Study the drawing (mm; zero at the part's minimum x, y, z) and answer. Give positions to 0.01 mm unless a question says otherwise; leave off trailing zeros. Write each loop counter-clockwise with the first axis right and the second up, starting at its lowest first coordinate (ties: lowest second). Pieces come first, ordered by that corner, then holes. Notation, with made-up numbers: (12, -6) - (57, -6) arc R17 ccw to (57, 3) - close; hole circle Ø11 at (76.25, 57). An arc over 180 degrees is marked (long way). Answer as CSV lines item,"result".
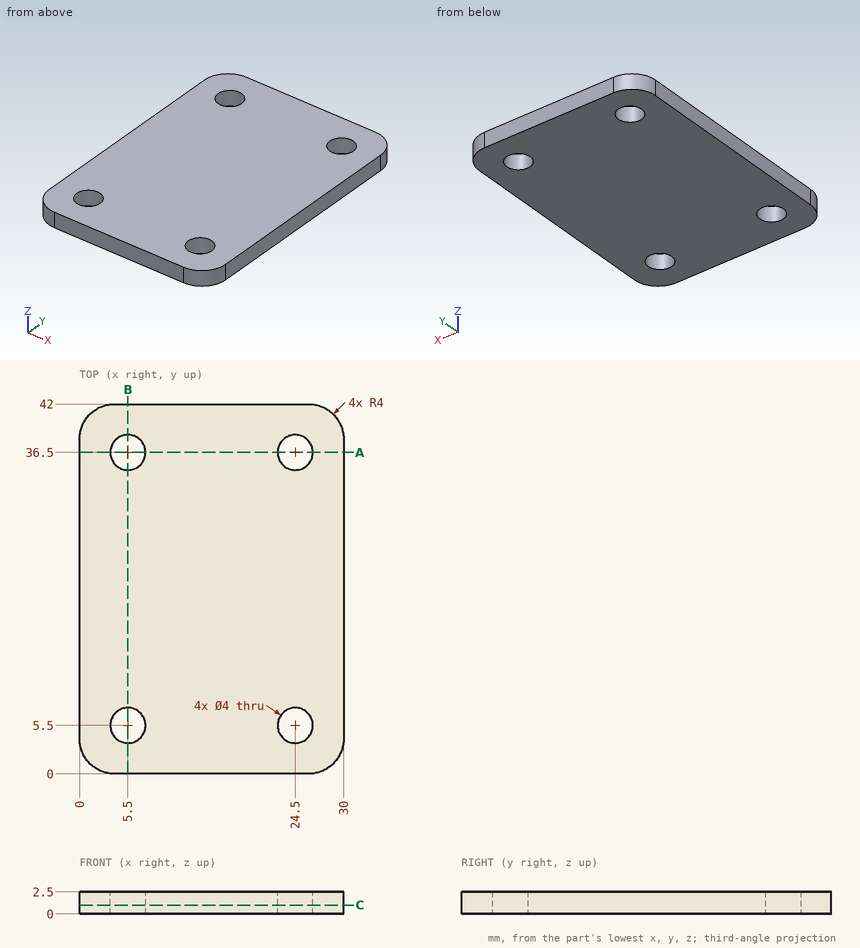
(1) A cutting plane is placed at A-A (y = 36.5). Write down the section's boundary in (x, z), and give its area (3 significant figures).
Worked out:
outline,"(0, 0) - (3.5, 0) - (3.5, 2.5) - (0, 2.5) - close; (7.5, 0) - (22.5, 0) - (22.5, 2.5) - (7.5, 2.5) - close; (26.5, 0) - (30, 0) - (30, 2.5) - (26.5, 2.5) - close"
area,"55.0 mm^2"
(2) Find the intervals of material crossed by L1, parallel to Y at x = 5.5, z = 1.6; L2, parallel to Y at x = 23.5, z = 1.4; L3, parallel to X at y = 6, z = 2.3, in increasing order.
Worked out:
L1,"y = 0 to 3.5, 7.5 to 34.5, 38.5 to 42"
L2,"y = 0 to 3.77, 7.23 to 34.77, 38.23 to 42"
L3,"x = 0 to 3.56, 7.44 to 22.56, 26.44 to 30"
(3) A cutting plane is placed at C-C (z = 1). Write down the section's boundary in (x, y), and give its area (3 significant figures).
Worked out:
outline,"(0, 4) arc R4 ccw to (4, 0) - (26, 0) arc R4 ccw to (30, 4) - (30, 38) arc R4 ccw to (26, 42) - (4, 42) arc R4 ccw to (0, 38) - close; hole circle Ø4 at (5.5, 5.5); hole circle Ø4 at (5.5, 36.5); hole circle Ø4 at (24.5, 5.5); hole circle Ø4 at (24.5, 36.5)"
area,"1,200 mm^2"
(4) A cutting plane is placed at B-B (x = 5.5). Write down the section's boundary in (y, z), and give its area (3 significant figures).
Worked out:
outline,"(0, 0) - (3.5, 0) - (3.5, 2.5) - (0, 2.5) - close; (7.5, 0) - (34.5, 0) - (34.5, 2.5) - (7.5, 2.5) - close; (38.5, 0) - (42, 0) - (42, 2.5) - (38.5, 2.5) - close"
area,"85.0 mm^2"
(5) This flat-tipped pin is pushed along its axis until it touches: P1, Ø2.5, axis at x = 5.5, y = 36.5, coming from the -Z side. Where does it stop, or does it pass through?
Worked out:
P1,"passes through"
